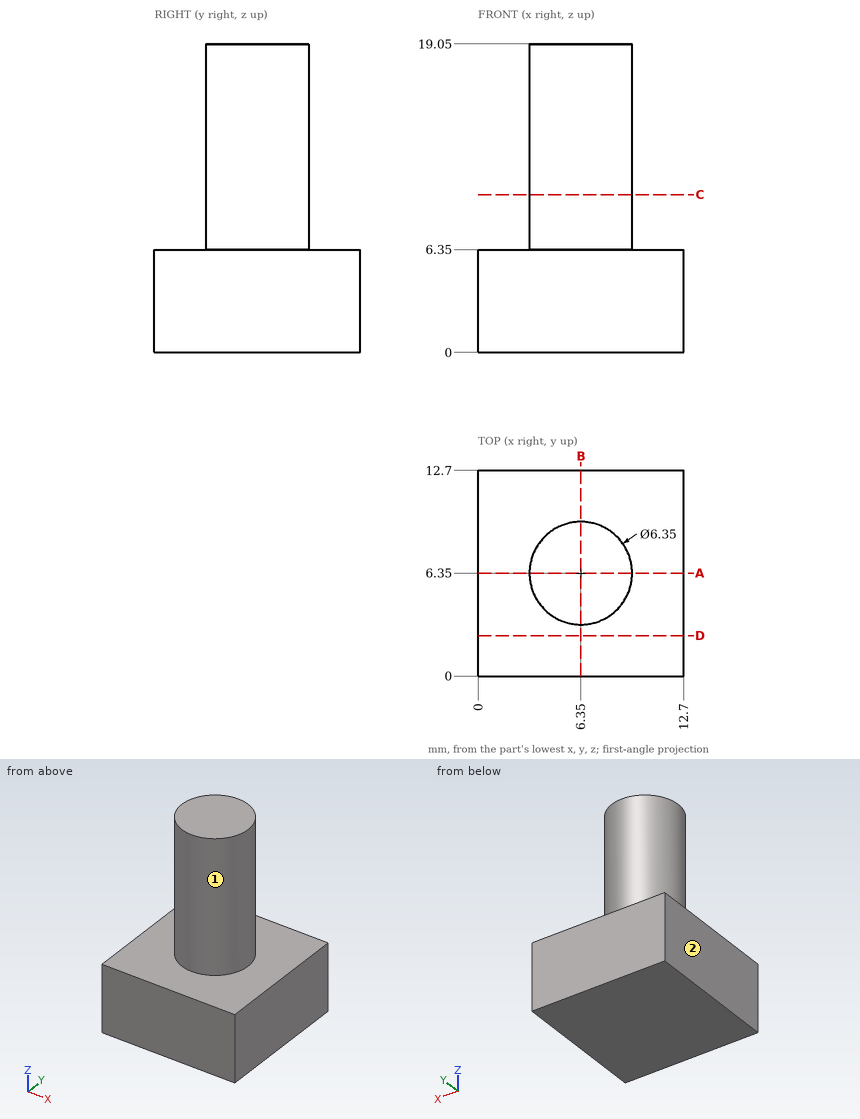
The figure shows three views and two pictorial views of one solid part (mm, origin at its lowest corner). Answer the questions. A direction names the side the tool comes from. Coordinates: 2 decimals unless noted, no trailing zeros. Loops run counter-clockwise (first coordinate to the right, second up) from the corner with the lowest first, then second, coordinate; pieces in that order, holes last. Notation, with made-up numbers: (11.25, -30.5) - (21.25, -30.5) arc R20 ccw to (21.25, -21.5) - close; hole circle Ø1 at (42, -24.5). An arc over 180 degrees is marked (long way). Use a Markdown table: item, result. Add a question column.
1) For the marked faces 1 and 2, determine the directions among +Z, -Z, +X, -X, +Y, -Y from which every point of the face is accessible in a straight line to the end or side of a thin tool.
2) Find the intervals of material crossed by line 1 (Z direction, x = 1, y = 4); line 2 (X direction, y = 6.25, z = 16); line 3 (Y direction, x = 8.25, z = 17.5), in increasing order.
3) Given pin 1 (1.5 mm diameter, centred on y = 9, z = 9, fed in from -X); pin 2 (3 mm diameter, centred on x = 10.5, y = 11, fed in from -Z); pin 3 (3 mm diameter, centred on x = 5.5, z = 10.5, fed in from -Y) (3 decimals), each flat-ended and moving along its own axis, determine where each tip first touches the part or whether it passes through.
4) The part is cut by section A-A, the plane y = 6.35. Give the vertices of the cut face in (x, z) (3 decimals), and give its area (3 significant figures).
5) The part is cut by section C-C, the plane z = 9.75. Give the vertices of the cut face in (x, y) (3 decimals), and give its area (3 significant figures).
6) The part is cut by section D-D, the plane y = 2.5. Give the vertices of the cut face in (x, z), and give its area (3 significant figures).
Here are the results:
| question | item | result |
|---|---|---|
| 1 | face 1 | +Z |
| 1 | face 2 | +Z, -Z, -X, +Y, -Y |
| 2 | line 1 | z = 0 to 6.35 |
| 2 | line 2 | x = 3.18 to 9.52 |
| 2 | line 3 | y = 3.81 to 8.89 |
| 3 | pin 1 | stops at x = 3.81 |
| 3 | pin 2 | stops at z = 0 |
| 3 | pin 3 | stops at y = 3.175 |
| 4 | outline | (0, 0) - (12.7, 0) - (12.7, 6.35) - (9.525, 6.35) - (9.525, 19.05) - (3.175, 19.05) - (3.175, 6.35) - (0, 6.35) - close |
| 4 | area | 161 mm^2 |
| 5 | outline | circle Ø6.35 at (6.35, 6.35) |
| 5 | area | 31.7 mm^2 |
| 6 | outline | (0, 0) - (12.7, 0) - (12.7, 6.35) - (0, 6.35) - close |
| 6 | area | 80.6 mm^2 |
